```python
from build123d import *

# Parameters (mm, degrees)
SKETCH_1_R             = 4.5
SKETCH_1_R_2           = 4
EXTRUDE_1_DEPTH        = 1.5
EXTRUDE_1_DEPTH_BACK   = 1.5
SKETCH_1_R_3           = 3
SKETCH_1_R_4           = 2.5
EXTRUDE_1_2_DEPTH      = 1.5
EXTRUDE_1_2_DEPTH_BACK = 1.5
SKETCH_2_R             = 4
SKETCH_2_R_2           = 3
EXTRUDE_2_DEPTH        = 1.2
EXTRUDE_2_DEPTH_BACK   = 1.2
SKETCH_3_R             = 5.1
SKETCH_3_R_2           = 4.5
EXTRUDE_3_DEPTH        = 0.6


with BuildPart() as part:
    # Sketch 1 → Extrude 1 (new body, two sides)
    with BuildSketch(Plane(origin=(0, 0, 0), x_dir=(1, 0, 0), z_dir=(0, 1, 0))) as extrude_1_sk:
        Circle(SKETCH_1_R)
        Circle(SKETCH_1_R_2, mode=Mode.SUBTRACT)
    extrude(amount=EXTRUDE_1_DEPTH)
    extrude(extrude_1_sk.sketch, amount=-EXTRUDE_1_DEPTH_BACK)



with BuildPart() as body_2:
    # Sketch 1 → Extrude 1 2 (new body, two sides)
    with BuildSketch(Plane(origin=(0, 0, 0), x_dir=(1, 0, 0), z_dir=(0, 1, 0))) as extrude_1_2_sk:
        Circle(SKETCH_1_R_3)
        Circle(SKETCH_1_R_4, mode=Mode.SUBTRACT)
    extrude(amount=EXTRUDE_1_2_DEPTH)
    extrude(extrude_1_2_sk.sketch, amount=-EXTRUDE_1_2_DEPTH_BACK)


with BuildPart() as part_1:
    add(part.part)

    add(body_2.part)  # Extrude 2 merges body 2
    # Sketch 2 → Extrude 2 (add, two sides)
    with BuildSketch(Plane(origin=(0, 0, 0), x_dir=(1, 0, 0), z_dir=(0, 1, 0))) as extrude_2_sk:
        Circle(SKETCH_2_R)
        Circle(SKETCH_2_R_2, mode=Mode.SUBTRACT)
    extrude(amount=EXTRUDE_2_DEPTH)
    extrude(extrude_2_sk.sketch, amount=-EXTRUDE_2_DEPTH_BACK)

    # Sketch 3 → Extrude 3 (add)
    with BuildSketch(Plane(origin=(0, 1.5, 0), x_dir=(1, 0, 0), z_dir=(0, 1, 0))):
        Circle(SKETCH_3_R)
        Circle(SKETCH_3_R_2, mode=Mode.SUBTRACT)
    extrude(amount=-EXTRUDE_3_DEPTH)


solid = part_1.part
```
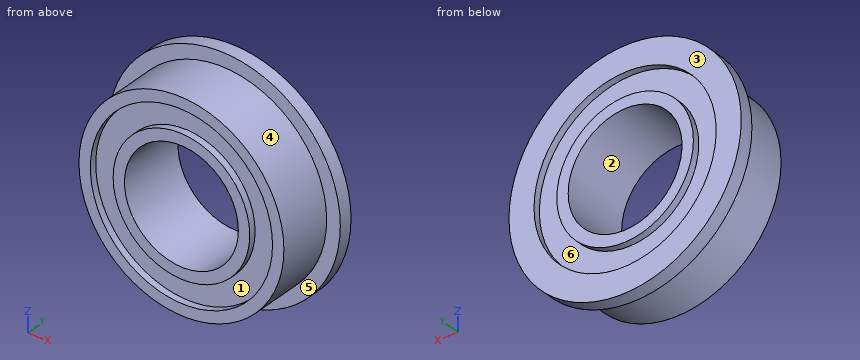
For this review, take the finished solid that the model builds, in its own axes (mm). Face numbers are marked on the shaded views. A direction names the side the tool comes from. Coordinates: 2 decimals unless noted, no trailing zeros. Write each loop counter-clockwise with the first axis right and the second up, starting at its lowest first coordinate (ties: lowest second). Pieces come first, ordered by that corner, then holes. Notation, with made-up numbers: (7, 79.25) - (46, 79.25) arc R21 ccw to (46, 90.25) - close; hole circle Ø3 at (-9, -32.75). An arc over 180 degrees is marked (long way). Answer in a Markdown table with one row per item. Add a question column.
Q1. For probe 1 along Z at (x, y) = (0, 1.35); probe 2 along X at (y, z) = (-1.3, 0), list the stretches that pass through material, from the lowest coordinate up.
Q2. We need section A-A, the plane x = 0. State the section outline as (y, z) points, and give its area (3 significant figures).
Q3. Tool access review of the marked faces 5 and 6: name each direction out of +Z, -Z, +X, -X, +Y, -Y from which nothing blocks a thin tool from reaching the whole face with its end or side.
Q4. We need section B-B, the plane z = -1.5. State the section outline as (x, y) points.
Q5. For P1, Ø6, axis at x = 0, z = 0, coming from the -Y side; P2, Ø1.5, axis at x = 2, y = -0.5, coming from the +Z side; P3, Ø1, axis at y = 1, z = 1, coming from the +X side; P4, Ø1, axis at y = 0, z = -1.5, coming from the -X side, all flat-tipped, find the tip position at first contact; note any pin that passes through.
Q6. Draft analysis for pull direction Z (two halves, no side actions). For the marked faces 1, 2, 3 and 4, state which applies: +Z half, -Z half, draft (parallel to the pull), parting line (faces both ways), or undercut.
Q7. We need section C-C, the plane y = -1.05. State the section outline as (x, z) points, and give its area (3 significant figures).
Q8. We need section D-D, the plane z = -3.5. State the section outline as (x, y) points, and give its area (3 significant figures).
Answer list:
| question | item | result |
|---|---|---|
| 1 | probe 1 | z = -5.1 to -4, -3 to -2.5, 2.5 to 3, 4 to 5.1 |
| 1 | probe 2 | x = -4.5 to -4, -3 to -2.5, 2.5 to 3, 4 to 4.5 |
| 2 | outline | (-1.5, -4.5) - (0.9, -4.5) - (0.9, -5.1) - (1.5, -5.1) - (1.5, -4) - (1.2, -4) - (1.2, -3) - (1.5, -3) - (1.5, -2.5) - (-1.5, -2.5) - (-1.5, -3) - (-1.2, -3) - (-1.2, -4) - (-1.5, -4) - close; (-1.5, 2.5) - (1.5, 2.5) - (1.5, 3) - (1.2, 3) - (1.2, 4) - (1.5, 4) - (1.5, 5.1) - (0.9, 5.1) - (0.9, 4.5) - (-1.5, 4.5) - (-1.5, 4) - (-1.2, 4) - (-1.2, 3) - (-1.5, 3) - close |
| 2 | area | 11.5 mm2 |
| 3 | face 5 | -Y |
| 3 | face 6 | +Y |
| 4 | outline | (-4.87, 0.9) - (-4.24, 0.9) - (-4.24, -1.5) - (-3.71, -1.5) - (-3.71, -1.2) - (-2.6, -1.2) - (-2.6, -1.5) - (-2, -1.5) - (-2, 1.5) - (-2.6, 1.5) - (-2.6, 1.2) - (-3.71, 1.2) - (-3.71, 1.5) - (-4.87, 1.5) - close; (2, -1.5) - (2.6, -1.5) - (2.6, -1.2) - (3.71, -1.2) - (3.71, -1.5) - (4.24, -1.5) - (4.24, 0.9) - (4.87, 0.9) - (4.87, 1.5) - (3.71, 1.5) - (3.71, 1.2) - (2.6, 1.2) - (2.6, 1.5) - (2, 1.5) - close |
| 5 | P1 | stops at y = -1.5 |
| 5 | P2 | stops at z = 4.32 |
| 5 | P3 | stops at x = 5.08 |
| 5 | P4 | stops at x = -4.39 |
| 6 | face 1 | undercut |
| 6 | face 2 | undercut |
| 6 | face 3 | draft |
| 6 | face 4 | parting line |
| 7 | outline | circle Ø9 at (0, 0); hole circle Ø5 at (0, 0) |
| 7 | area | 44.0 mm2 |
| 8 | outline | (-3.71, 0.9) - (-2.83, 0.9) - (-2.83, -1.5) - (-1.94, -1.5) - (-1.94, -1.2) - (1.94, -1.2) - (1.94, -1.5) - (2.83, -1.5) - (2.83, 0.9) - (3.71, 0.9) - (3.71, 1.5) - (1.94, 1.5) - (1.94, 1.2) - (-1.94, 1.2) - (-1.94, 1.5) - (-3.71, 1.5) - close |
| 8 | area | 15.7 mm2 |
